For this review, use the dimensioned drawing (mm, ordinates from the lowest corner) and the shaded views. Coordinates: 2 decimals unless noted, no trailing zeros. Order: outer loops, then holes, each group sorted by start corner. A loop starts at its lowest first (then second) coordinate and runs counter-clockwise, first axis right, second up. Notation, with made-up numbers: M 89.25,13.25 L 118.25,13.25 A18 cw 118.25,24.25 Z; hole C 63,45.25 d2. An arc over 180 degrees is marked long. One line per item, written item: value.
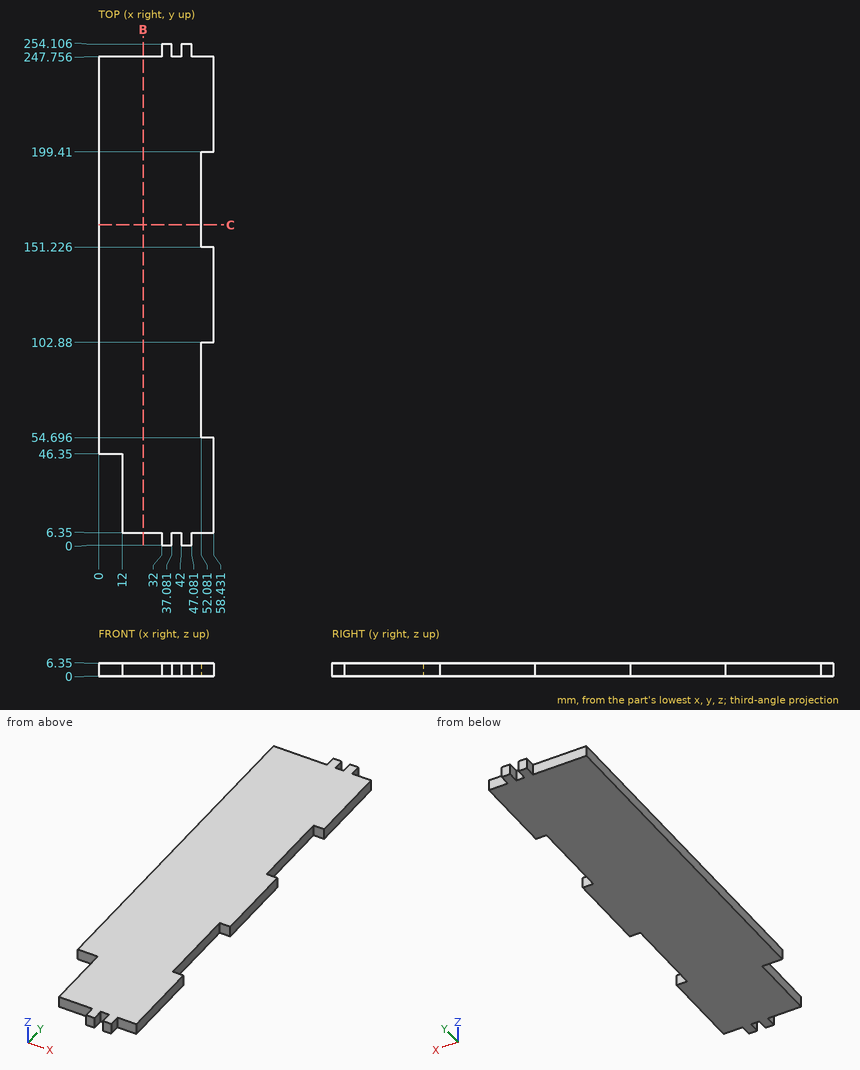
(1) We need section C-C, the plane y = 162.5. State the section outline as (x, z) points, plus the area to 3 significant figures.
Geometry results:
outline: M 0,0 L 52.08,0 L 52.08,6.35 L 0,6.35 Z
area: 331 mm2
(2) Insertion check: pin 1 Ø3 at (x, z) = (29, 2.5) entering from -Y; pin 2 Ø3 at (y, z) = (4.5, 1.5) entering from +X; pin 3 Ø3 at (y, z) = (250.5, 4.5) entering from -X; pin 4 Ø10 at (x, y) = (8, 63.5) entering from -Z. Each pin has a flat end and moves straight along its axis. Give the tip position at first contact, or say it passes through.
Geometry results:
pin 1: stops at y = 6.35
pin 2: stops at x = 47.08
pin 3: stops at x = 32
pin 4: stops at z = 0
(3) We need section B-B, the plane x = 22.5. State the section outline as (y, z) points, plus the area to 3 significant figures.
Geometry results:
outline: M 6.35,0 L 247.76,0 L 247.76,6.35 L 6.35,6.35 Z
area: 1,530 mm2
(4) For L1, parallel to Y at x = 55, z = 6; L2, parallel to Y at x = 15.5, z = 1.75; L3, parallel to X at y = 157, z = 2.25, list the stretches that pass through material, from the lowest coordinate up.
Geometry results:
L1: y = 6.35 to 54.7, 102.88 to 151.23, 199.41 to 247.76
L2: y = 6.35 to 247.76
L3: x = 0 to 52.08
